```python
from build123d import *

# Parameters (mm, degrees)
F0_R       = 51.4602695285
F1_DEPTH   = 25.4
F2_DEPTH   = 28.956
F3_R       = 17.858664642
F3_R_2     = 19.3013042732
F1_FACE1_R = 51.4602695285
F4_DEPTH   = 59.182
F5_R       = 8.4878937559
F6_DEPTH   = 35.5


with BuildPart() as f1:
    # F0 (on Top) → F1 (new body)
    with BuildSketch(Plane.XY):
        Circle(F0_R)
    extrude(amount=F1_DEPTH)

    # F2 (add): a face of the model
    f2_faces = [f1.faces().sort_by_distance(p)[0] for p in [
        (0, 0, 25.4),
    ]]
    extrude(f2_faces, amount=F2_DEPTH)

    # F3 (on Top) + F1_face1 (on face) → F4 (join)
    with BuildSketch(Plane.XY):
        with Locations((44.8872148991, 51.7368838191)):
            Circle(F3_R)
        with Locations((-47.2190156579, 51.7368838191)):
            Circle(F3_R_2)
    with BuildSketch(Plane(origin=(0, 0, 0), x_dir=(1, 0, 0), z_dir=(0, 0, -1))):
        Circle(F1_FACE1_R)
    extrude(amount=F4_DEPTH, dir=(0, 0, 1))

    # F5 (on Top) → F6 (cut)
    with BuildSketch(Plane.XY):
        with Locations((-37.1631160378, 0)):
            Circle(F5_R)
        with Locations((-26.2782913604, 26.2782913604)):
            Circle(F5_R)
        with Locations((0, 37.1631160378)):
            Circle(F5_R)
        with Locations((26.2782913604, 26.2782913604)):
            Circle(F5_R)
        with Locations((37.1631160378, 0)):
            Circle(F5_R)
        with Locations((26.2782913604, -26.2782913604)):
            Circle(F5_R)
        with Locations((0, -37.1631160378)):
            Circle(F5_R)
        with Locations((-26.2782913604, -26.2782913604)):
            Circle(F5_R)
    extrude(amount=F6_DEPTH, mode=Mode.SUBTRACT)


solid = f1.part
```
The listing builds one solid part. Answer for the finished solid, in the listing's coordinates (mm). A direction names the side the tool comes from. Coordinates: 2 decimals unless noted, no trailing zeros. Write each loop counter-clockwise with the first axis right and the second up, starting at its lowest first coordinate (ties: lowest second). Pieces come first, ordered by that corner, then holes. Notation, with made-up numbers: (83, 20) - (94, 20) arc R23 ccw to (94, 32) - close; hole circle Ø3 at (12, -36). An arc over 180 degrees is marked (long way). Return JSON: item names as keys, results as strings. Group by question number.
1. Given pin 1 (4 mm diameter, centred on x = 21.5, z = 16, fed in from +Y); pin 2 (8.5 mm diameter, centred on x = -0.5, y = 38.5, fed in from -Z); pin 3 (18.5 mm diameter, centred on x = -22, y = -23.5, fed in from -Z); pin 4 (2 mm diameter, centred on y = 44, z = 53, fed in from -X), each flat-ended and moving along its own axis, determine where each tip first touches the part or whether it passes through.
2. Determine the mould class of faces 1 (the flat face through (-3, 11, 59.182)), 2 (the cylindrical face through (30.427, -5.165, 17.502)) for opening direction X: released by +X, released by -X, zero draft, split by the parting line, or undercut.
3. A cutting plane is placed at A-A, the plane x = 0. Determine the outline of the cut face in (y, z).
4. A cutting plane is placed at D-D, the plane x = 39. Determine the outline of the cut face in (y, z), plus the area to 3 significant figures.
5. A cutting plane is placed at C-C, the plane z = 28.5. Give the number of separate pieces and of enclosed holes in the cut face, plus the area to 3 significant figures.
6. Which of the six approach directions +Z, -Z, +X, -X, +Y, -Y give full straight-line access (tool end or side, diameter ignored) to faces 3 (the cylindrical face through (-1.84, -45.45, 17.5)), 4 (the flat face through (-3, 11, 0))?
7. Straight lines are drawn through the part: L1, parallel to Y at x = 0.5, z = 29.5; L2, parallel to Y at x = 0, z = 14.5. For each, find the intervals that lie inside material, in ascending order.
Ans:
{
 "1": {"pin 1": "y = 47.62", "pin 2": "z = 35.5", "pin 3": "z = 0", "pin 4": "x = -65.31"},
 "2": {"face 1": "zero draft", "face 2": "undercut"},
 "3": {"outline": "(-51.46, 0) - (-45.65, 0) - (-45.65, 35.5) - (-28.68, 35.5) - (-28.68, 0) - (28.68, 0) - (28.68, 35.5) - (45.65, 35.5) - (45.65, 0) - (51.46, 0) - (51.46, 59.18) - (-51.46, 59.18) - close"},
 "4": {"outline": "(-33.57, 0) - (-8.29, 0) - (-8.29, 35.5) - (8.29, 35.5) - (8.29, 0) - (33.57, 0) - (33.57, 59.18) - (-33.57, 59.18) - close; (34.88, 0) - (68.6, 0) - (68.6, 59.18) - (34.88, 59.18) - close", "area": "5,380 mm²"},
 "5": {"separate pieces": "1", "enclosed holes": "8", "area": "8,670 mm²"},
 "6": {"face 3": "-Z", "face 4": "-Z, +X, -X, +Y, -Y"},
 "7": {"L1": "-51.46 to -45.64, -28.69 to 28.69, 45.64 to 51.46", "L2": "-51.46 to -45.65, -28.68 to 28.68, 45.65 to 51.46"}
}
